from build123d import *

# Parameters (mm, degrees)
F1_DEPTH     = 10
F2_DEPTH     = 10
F3_R         = 5
F4_T1_DEPTH  = 71.883894651
F5_T1_DEPTH  = 56.6843134125
F6_SIZE      = 3
F7_SIZE      = 5
F10_DEPTH    = 10
F9_W         = 35
F9_H         = 2
F11_DEPTH    = 10
F12_T4_DEPTH = 157.651683953
F13_T4_DEPTH = 157.651683953
F14_W        = 8
F14_H        = 2
F15_W        = 8
F15_H        = 2
F16_DEPTH    = 15
F17_SIZE2    = 4.6630765815
F17_SIZE     = 10
F18_SIZE2    = 4.6630765815
F18_SIZE     = 10
F19_R        = 0.99999
F20_R        = 5
F21_DEPTH    = 45
F22_R        = 2.9781353661
F23_DEPTH    = 5
F25_W        = 2
F25_H        = 2
F26_DEPTH    = 4
F28_DEPTH    = 15
F29_DEPTH    = 5
F30_W        = 5
F30_H        = 2
F31_DEPTH    = 2
F32_SIZE     = 3
F33_R        = 0.99999


# Not quite as in the source:
# - a fillet or chamfer that OpenCascade refuses, or shapes differently, is made with other operations: its cross-section is extruded or revolved along the edge and cut away or added
# - a fillet or chamfer is up to 0.001 mm smaller than in the source, because OpenCascade refuses the exact size


with BuildPart() as f1:
    # F0 (on Right) → F1 (new body)
    with BuildSketch(Plane.YZ):
        Polygon((30, 5), (30, 0), (44.9290536344, 5), (9.4593074173, 11.7742568254), (-1.5650746645, 11.7742568254), (-11.31126564, 5), align=None)
        Polygon((30, 0), (0, 0), (-30, 0), (-30, -5), (30, -5), align=None)
        Polygon((-30, 0), (0, 0), (30, 0), (30, 5), (-11.31126564, 5), (-30, 5), align=None)
    extrude(amount=-F1_DEPTH)

    # F2 (add): a face of the model
    f2_faces = [f1.faces().sort_by_distance(p)[0] for p in [
        (0, 4.6213303299, 2.1526362718),
    ]]
    extrude(f2_faces, amount=F2_DEPTH)

    # F3
    f3_edges = [f1.edges().sort_by_distance(p)[0] for p in [
        (-10, -6.43817, 8.387128),
        (10, -6.43817, 8.387128),
    ]]
    fillet(f3_edges, radius=F3_R)

    # F4: chamfer of 10 x 3.6397023427 on 1 edges, made by hand

    # F4_s2 → F4_t1 (cut)
    with BuildSketch(Plane.YZ.offset(-35.9419473255)):
        Polygon((-20, 5), (-30, 1.3602976573), (-30, 5), align=None)
    extrude(amount=F4_T1_DEPTH, mode=Mode.SUBTRACT)

    # F5: chamfer of 2 on 2 edges, made by hand

    # F5_s2 → F5_t1 (cut)
    with BuildSketch(Plane(origin=(0, 47.4786197454, -9.0677943367), x_dir=(1, 0, 0), z_dir=(0, -0.9822462418, 0.1875961634))):
        Polygon((-10, 11.3397492965), (-8, 13.3397492965), (-10, 13.3397492965), align=None)
        Polygon((10, 11.3397492965), (8, 13.3397492965), (10, 13.3397492965), align=None)
    extrude(amount=F5_T1_DEPTH, mode=Mode.SUBTRACT)

    # F6
    f6_edges = [f1.edges().sort_by_distance(p)[0] for p in [
        (0, 30, -5),
    ]]
    chamfer(f6_edges, length=F6_SIZE)

    # F7
    f7_edges = [f1.edges().sort_by_distance(p)[0] for p in [
        (-10, -30, -1.819851),
        (10, -30, -1.819851),
    ]]
    chamfer(f7_edges, length=F7_SIZE)

    # F8 (on face) → F10 (join)
    with BuildSketch(Plane.YZ.offset(10)):
        Polygon((-13, 0), (0, 0), (22, 0), (22, 2), (-13, 2), align=None)
    extrude(amount=F10_DEPTH)

    # F9 (on face) → F11 (join)
    with BuildSketch(Plane(origin=(-10, 0, 0), x_dir=(0, -1, 0), z_dir=(-1, 0, 0))):
        with Locations((-4.5269672573, 1)):
            Rectangle(F9_W, F9_H)
    extrude(amount=F11_DEPTH)

    # F12: chamfer of 30 x 10.919107028 on 1 edges, made by hand


with BuildPart() as f12_tool2:
    # F12_s3 → F12_t4 (new body)
    with BuildSketch(Plane.XY.offset(-77.8258419765)):
        Polygon((-9.080892972, -12.9730327427), (-20, 17.0269672573), (-20, -12.9730327427), align=None)
    extrude(amount=F12_T4_DEPTH)

    split(bisect_by=Plane.YZ.offset(-10), keep=Keep.BOTTOM)


with BuildPart() as f1_1:
    add(f1.part)

    # F12_t1: cut F12_tool2
    add(f12_tool2.part, mode=Mode.SUBTRACT)

    # F13: chamfer of 30 x 10.919107028 on 1 edges, made by hand


with BuildPart() as f13_tool2:
    # F13_s3 → F13_t4 (new body)
    with BuildSketch(Plane.XY.offset(79.8258419765)):
        Polygon((9.080892972, -13), (20, 17), (20, -13), align=None)
    extrude(amount=-F13_T4_DEPTH)

    split(bisect_by=Plane.YZ.offset(10), keep=Keep.TOP)


with BuildPart() as f1_2:
    add(f1_1.part)

    # F13_t1: cut F13_tool2
    add(f13_tool2.part, mode=Mode.SUBTRACT)

    # F14 (on face) + F15 (on face) → F16 (join)
    with BuildSketch(Plane(origin=(0, 22, 0), x_dir=(-1, 0, 0), z_dir=(0, 1, 0))):
        with Locations((-16, 1)):
            Rectangle(F14_W, F14_H)
    with BuildSketch(Plane(origin=(0, 22.0269672573, 0), x_dir=(-1, 0, 0), z_dir=(0, 1, 0))):
        with Locations((16, 1)):
            Rectangle(F15_W, F15_H)
    extrude(amount=F16_DEPTH)

    # F17
    f17_edges = [f1_2.edges().sort_by_distance(p)[0] for p in [
        (20, 37, 1),
    ]]
    f17_side = f1_2.faces().sort_by_distance((20, 27, 1))[0]
    chamfer(f17_edges, length=F17_SIZE, length2=F17_SIZE2, reference=f17_side)

    # F18
    f18_edges = [f1_2.edges().sort_by_distance(p)[0] for p in [
        (-20, 37.026967, 1),
    ]]
    f18_side = f1_2.faces().sort_by_distance((-20, 27.026967, 1))[0]
    chamfer(f18_edges, length=F18_SIZE, length2=F18_SIZE2, reference=f18_side)

    # F19 (radius 1 in the source; OpenCascade refuses exactly that, so slightly less here)
    f19_edges = [f1_2.edges().sort_by_distance(p)[0] for p in [
        (15, 3.262613, 2),
        (15, 3.262613, 0),
        (17.668462, 32, 0),
        (17.668462, 32, 2),
        (12, 29.5, 2),
        (12, 29.5, 0),
        (-15, 3.28958, 2),
        (-15, 3.28958, 0),
        (-17.668462, 32.026967, 2),
        (-12, 29.526967, 2),
        (-12, 29.526967, 0),
    ]]
    fillet(f19_edges, radius=F19_R)

    # F20 (on Front) → F21 (join)
    with BuildSketch(Plane.XZ):
        with Locations((0, 2.7116553392)):
            Circle(F20_R)
    extrude(amount=-F21_DEPTH)

    # F22 (on face) → F23 (cut)
    with BuildSketch(Plane(origin=(0, 45, 0), x_dir=(-1, 0, 0), z_dir=(0, 1, 0))):
        with Locations((0, 2.7116553392)):
            Circle(F22_R)
    extrude(amount=-F23_DEPTH, mode=Mode.SUBTRACT)

    # F24: chamfer of 2 on 1 edges, made by hand


with BuildPart() as f24_tool2:
    # F24_s3 → F24_t4 (revolve)
    with BuildSketch(Plane.XY.offset(2.7116553392)):
        Polygon((5, 43), (3, 45), (5, 45), align=None)
    revolve(axis=Axis((0, 45, 2.7116553392), (0, -1, 0)))

    split(bisect_by=Plane(origin=(0, 3.0256985599, -9.0341632165), x_dir=(1, 0, 0), z_dir=(0, 0.3175793108, -0.9482317129)), keep=Keep.TOP)


with BuildPart() as f1_3:
    add(f1_2.part)

    # F24_t1: cut F24_tool2
    add(f24_tool2.part, mode=Mode.SUBTRACT)


with BuildPart() as f24_tool7:
    # F24_s8 → F24_t9 (revolve)
    with BuildSketch(Plane.XY.offset(2.7116553392)):
        Polygon((5, 43), (3, 45), (5, 45), align=None)
    revolve(axis=Axis((0, 45, 2.7116553392), (0, -1, 0)))

    split(bisect_by=Plane(origin=(0, 2.5024857889, 13.1029186126), x_dir=(1, 0, 0), z_dir=(0, 0.1875961634, 0.9822462418)), keep=Keep.TOP)


with BuildPart() as f1_4:
    add(f1_3.part)

    # F24_t6: cut F24_tool7
    add(f24_tool7.part, mode=Mode.SUBTRACT)

    # F25 (on face) → F26 (join)
    with BuildSketch(Plane(origin=(0, 2.5024857889, 13.1029186126), x_dir=(1, 0, 0), z_dir=(0, 0.1875961634, 0.9822462418))):
        with Locations((-6, 39.4243540466)):
            Rectangle(F25_W, F25_H)
        with Locations((6, 39.4243540466)):
            Rectangle(F25_W, F25_H)
    extrude(amount=F26_DEPTH)

    # F27 (on face) → F28 (join)
    with BuildSketch(Plane(origin=(5, 0, 0), x_dir=(0, -1, 0), z_dir=(-1, 0, 0))):
        Polygon((-42.9595402808, 9.4484498521), (-40.9950477973, 9.8236421789), (-45.9950477973, 9.8236421789), (-45.9950477973, 7.8236421789), (-42.6492233025, 7.8236421789), align=None)
        Polygon((-40.9950477973, 7.8236421789), (-40.9950477973, 9.8236421789), (-42.9595402808, 9.4484498521), (-42.6492233025, 7.8236421789), align=None)
    extrude(amount=F28_DEPTH)

    # F27 (on face) → F29 (join)
    with BuildSketch(Plane(origin=(5, 0, 0), x_dir=(0, -1, 0), z_dir=(-1, 0, 0))):
        Polygon((-42.9595402808, 9.4484498521), (-40.9950477973, 9.8236421789), (-45.9950477973, 9.8236421789), (-45.9950477973, 7.8236421789), (-42.6492233025, 7.8236421789), align=None)
        Polygon((-40.9950477973, 7.8236421789), (-40.9950477973, 9.8236421789), (-42.9595402808, 9.4484498521), (-42.6492233025, 7.8236421789), align=None)
    extrude(amount=-F29_DEPTH)

    # F30 (on face) → F31 (join)
    with BuildSketch(Plane.XZ.offset(-40.9950477973)):
        with Locations((-7.5, 8.8236421789)):
            Rectangle(F30_W, F30_H)
        Polygon((-5, 7.8236421789), (0, 7.8236421789), (5, 7.8236421789), (5, 9.8236421789), (0, 9.8236421789), (-5, 9.8236421789), align=None)
        with Locations((7.5, 8.8236421789)):
            Rectangle(F30_W, F30_H)
    extrude(amount=F31_DEPTH)

    # F32
    f32_edges = [f1_4.edges().sort_by_distance(p)[0] for p in [
        (-10, 38.995048, 8.823642),
        (10, 38.995048, 8.823642),
    ]]
    chamfer(f32_edges, length=F32_SIZE)

    # F33 (radius 1 in the source; OpenCascade refuses exactly that, so slightly less here)
    f33_edges = [f1_4.edges().sort_by_distance(p)[0] for p in [
        (0, 38.995048, 7.823642),
        (0, 38.995048, 9.823642),
        (-8.5, 40.495048, 9.823642),
        (-8.5, 40.495048, 7.823642),
        (8.5, 40.495048, 9.823642),
        (8.5, 40.495048, 7.823642),
        (10, 43.995048, 7.823642),
        (10, 43.995048, 9.823642),
        (-10, 43.995048, 9.823642),
        (-10, 43.995048, 7.823642),
    ]]
    fillet(f33_edges, radius=F33_R)


solid = f1_4.part
For this review, take the finished solid that the model builds, in its own axes (mm). A direction names the side the tool comes from. Round coordinates to 2 decimals unless told otherwise and drop trailing zeros. Order: outer loops, then holes, each group sorted by start corner. A loop starts at its lowest first (then second) coordinate and runs counter-clockwise, first axis right, second up. Notation, with made-up numbers: (-34, 60.25) -> (14, 60.25) arc R33 cw to (14, 90.25) -> close; hole circle Ø9 at (-22, 41.25). An arc over 180 degrees is marked (long way). Put each result on its own line as item: value.
Q1. For probe 1 along Z at (x, y) = (14.5, 20); probe 2 along X at (y, z) = (17, 6.75); probe 3 along X at (y, z) = (-6, 6.5), list the stretches that pass through material, from the lowest coordinate up. Write a range as [from, to].
Check result:
probe 1: [0, 2]
probe 2: [-10, 10]
probe 3: [-8.84, 8.84]
Q2. Add section C-C on y = 34. State how many separate pieces and enclosed holes the cut face has, plus the area to 3 significant figures.
Check result:
separate pieces: 3
enclosed holes: 0
area: 156 mm2
Q3. Insertion check: pin 1 Ø3 at (x, z) = (-16, 2.5) entering from +Y; pin 2 Ø1.8 at (x, y) = (-1.5, 43) entering from -Z; pin 3 Ø5 at (x, y) = (3, 37) entering from +Z. Each pin has a flat end and moves straight along its axis. Give the tip position at first contact, or say it passes through.
Check result:
pin 1: y = 37.03
pin 2: z = -2.25
pin 3: z = 9.69
Q4. Add section D-D on y = -22. Write out the cut boundary in (x, z).
Check result:
outline: (-10, -5) -> (10, -5) -> (10, 4.27) -> (-10, 4.27) -> close
Q5. Add section B-B on y = -12.5. Write out the cut boundary in (x, z).
Check result:
outline: (-10, -5) -> (10, -5) -> (10, 5) -> (-10, 5) -> close
Q6. Machinability: for faces 1 (the flat face through (14, 14, 0)), 2 (the flat face through (-7, 41, 7)), 3 (the flat face through (14, 37, 1)), which of the approach directions +Z, -Z, +X, -X, +Y, -Y give a long, thin tool a straight path to every point of the face, cutting with its end or side? Answer none if there is none.
Check result:
face 1: -Z, +X, +Y, -Y
face 2: -X, +Y
face 3: +Z, -Z, +X, +Y
Q7. Mouldability with a two-part tool opening along Y and no side actions: class faces 4 (the cylindrical face through (-15.111, 4.473, 1.715)), 5 (the flat face through (14, 14, 2)), 6 (the flat face through (0, 28, -4)), 7 (the flat face through (-9.014, 24.016, 7.962)) as pulls with the +Y half, pulls with the -Y half, needs draft (parallel to the pull), parting line crosses it, or undercut.
Check result:
face 4: pulls with the -Y half
face 5: needs draft
face 6: pulls with the +Y half
face 7: undercut
